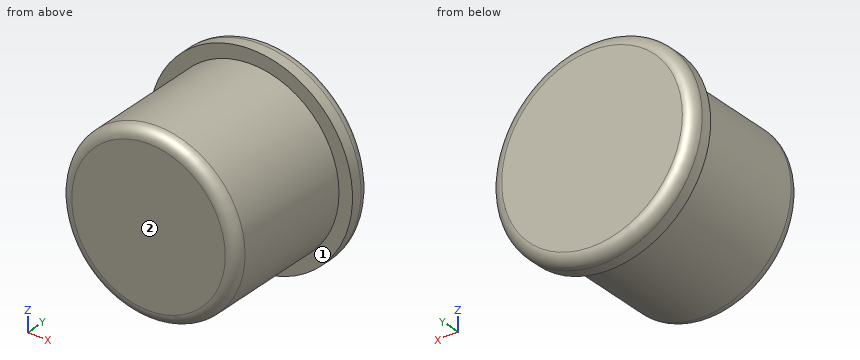
Autodesk Inventor part; units mm, degrees
ref_plane "YZ Plane" through (0, 0, 0) normal (1, 0, 0) x (0, 1, 0)
ref_plane "XZ Plane" through (0, 0, 0) normal (0, 1, 0) x (-1, 0, 0)
ref_plane "XY Plane" through (0, 0, 0) normal (0, 0, 1) x (1, 0, 0)
sketch "Boceto1" plane through (0, 0, 0) normal (0, 1, 0) x (-1, 0, 0)
  circle A0 centre (0, 0) radius 4.5
  dimension "d0" = 9
extrude "Extrusión1" add sketch "Boceto1" along normal blind 1
fillet "Empalme1" radius 0.5 1 edges at (4.5, 1, 0)
sketch "Boceto2" plane through (0, 0, 0) normal (0, -1, 0) x (1, 0, 0)
  circle A0 centre (0, 0) radius 3.9
  dimension "d4" = 7.8
extrude "Extrusión2" add sketch "Boceto2" along normal blind 6
fillet "Empalme2" radius 0.5 1 edges at (-3.9, -6, 0)
properties part number "sensor"
Verification items for the finished model (mm, model axes). Face numbers are marked on the shaded views. A direction names the side the tool comes from. Give positions to 0.01 mm unless a question says otherwise; leave off trailing zeros. Order: outer loops, then holes, each group sorted by start corner. A loop starts at its lowest first (then second) coordinate and runs counter-clockwise, first axis right, second up. Notation, with made-up numbers: M 60.5,-17 L 75.5,-17 A24 cw 75.5,1 Z; hole C 38,-10 d2. An arc over 180 degrees is marked long. Return JSON: item names as keys, results as strings. Group by question number.
1) Go/stop test with a flat-tipped pin: pin 1 Ø2 at (x, y) = (1, -4) entering from -Z. Record where the tip stops, or that it passes through.
2) Section check B-B on y = -0.75. Record the cut outline in (x, z).
3) Section check A-A on x = 0. Record the cut outline in (y, z), and give its area (3 significant figures).
4) Access from +Z, -Z, +X, -X, +Y, -Y to the whole of each face (thin tool, end or side, straight path). Record for the marked faces 1 and 2.
5) Scan lines: line 1 (Z direction, x = 0, y = -2.5); line 2 (Z direction, x = 2, y = -5.25); line 3 (Y direction, x = 3.5, z = -1). Record each from-to range of solid material in increasing order.
Answer block:
{
 "1": {"pin 1": "stops at z = -3.9"},
 "2": {"outline": "C 0,0 d7.8"},
 "3": {"outline": "M -6,-3.4 A0.5 ccw -5.5,-3.9 L 0,-3.9 L 0,-4.5 L 0.5,-4.5 A0.5 ccw 1,-4 L 1,4 A0.5 ccw 0.5,4.5 L 0,4.5 L 0,3.9 L -5.5,3.9 A0.5 ccw -6,3.4 Z", "area": "55.6 mm^2"},
 "4": {"face 1": "-Y", "face 2": "+Z, -Z, +X, -X, -Y"},
 "5": {"line 1": "z = -3.9 to 3.9", "line 2": "z = -3.35 to 3.35", "line 3": "y = -5.94 to 1"}
}
